Check sheet for the modelled part. Datum: model origin and axes. Units: mm. Face numbers are marked on the shaded views. Coordinates: 2 decimals unless noted, no trailing zeros. Loops run counter-clockwise (first coordinate to the right, second up) from the corner with the lowest first, then second, coordinate; pieces in that order, holes last. Notation, with made-up numbers: (47, 61.25) -> (102, 61.25) arc R15 ccw to (102, 79.25) -> close; hole circle Ø5 at (86, 3.5). An arc over 180 degrees is marked (long way). Use CSV: the item, a comma, the result in double quotes.
```python
from build123d import *
from OCP.BRepFilletAPI import BRepFilletAPI_MakeChamfer

# Parameters (mm, degrees)
BOSS_EXTRUDE1_DEPTH = 2.5
BOSS_EXTRUDE2_DEPTH = 5.5
CHAMFER2_SIZE       = 5.5
CHAMFER2_SIZE_2     = 0.192064232
CHAMFER3_SIZE       = 0.8
CHAMFER3_SIZE2      = 0.829452764


with BuildPart() as part:
    # Sketch1 → Boss-Extrude1 (new body)
    with BuildSketch(Plane(origin=(0, 0, 0), x_dir=(1, 0, 0), z_dir=(0, 1, 0))):
        with BuildLine():
            Line((-23, 17.5), (23, 17.5))
            ThreePointArc((23, 17.5), (28.656854249, 15.156854249), (31, 9.5))
            Line((31, 9.5), (31, -9.5))
            ThreePointArc((31, -9.5), (28.656854249, -15.156854249), (23, -17.5))
            Line((23, -17.5), (-23, -17.5))
            ThreePointArc((-23, -17.5), (-28.656854249, -15.156854249), (-31, -9.5))
            Line((-31, -9.5), (-31, 9.5))
            ThreePointArc((-31, 9.5), (-28.656854249, 15.156854249), (-23, 17.5))
        make_face()
    extrude(amount=BOSS_EXTRUDE1_DEPTH)

    # Sketch2 → Boss-Extrude2 (add)
    with BuildSketch(Plane(origin=(0, 2.5, 0), x_dir=(1, 0, 0), z_dir=(0, 1, 0))):
        with BuildLine():
            Line((-28.85, -7.8), (-28.85, 7.8))
            ThreePointArc((-28.85, 7.8), (-20.4, 16.25), (-11.95, 7.8))
            Line((-11.95, 7.8), (-11.95, -7.8))
            ThreePointArc((-11.95, -7.8), (-20.4, -16.25), (-28.85, -7.8))
        make_face()
        with BuildLine():
            Line((-8.45, -7.8), (-8.45, 7.8))
            ThreePointArc((-8.45, 7.8), (0, 16.25), (8.45, 7.8))
            Line((8.45, 7.8), (8.45, -7.8))
            ThreePointArc((8.45, -7.8), (0, -16.25), (-8.45, -7.8))
        make_face()
        with BuildLine():
            Line((11.95, -7.8), (11.95, 7.8))
            ThreePointArc((11.95, 7.8), (20.4, 16.25), (28.85, 7.8))
            Line((28.85, 7.8), (28.85, -7.8))
            ThreePointArc((28.85, -7.8), (20.4, -16.25), (11.95, -7.8))
        make_face()
    extrude(amount=BOSS_EXTRUDE2_DEPTH)

    # Chamfer2
    # the kernel refuses this chamfer: 5.5, 0.192064232 mm, written as the material it takes off along each edge
    with BuildSketch(Plane(origin=(-28.85, 8, 7.8), x_dir=(-0.0013423185755924486, -0.9999990990900149, 0), z_dir=(0, 0, -1))) as chamfer2_piece_1_section:
        Polygon((CHAMFER2_SIZE * 0.99999909909, -CHAMFER2_SIZE * 0.00134231857559), (-CHAMFER2_SIZE_2 * 0.00134231857702, -CHAMFER2_SIZE_2 * 0.999999100155), (0, 0), align=None)
    chamfer2_piece_1 = extrude(amount=15.6, mode=Mode.PRIVATE)
    chamfer2_piece_1 = split(chamfer2_piece_1, bisect_by=Plane(origin=(-28.848299171, 2.5, 0), z_dir=(0, 1, 0)), keep=Keep.TOP, mode=Mode.PRIVATE)
    add(chamfer2_piece_1, mode=Mode.SUBTRACT)
    with BuildSketch(Plane(origin=(-20.4, 8, -7.8), x_dir=(-1, 0, 0), z_dir=(0, 0, 1))) as chamfer2_piece_2_section:
        Polygon((8.45, CHAMFER2_SIZE), (8.45 - CHAMFER2_SIZE_2 * 1.00000000107, 0), (8.45, 0), align=None)
    chamfer2_piece_2 = revolve(axis=Axis((-20.4, 8, -7.8), (0, -1, 0)), revolution_arc=180, mode=Mode.PRIVATE)
    chamfer2_piece_2 = split(chamfer2_piece_2, bisect_by=Plane(origin=(-20.4, 2.5, -16.18152008), z_dir=(0, 1, 0)), keep=Keep.TOP, mode=Mode.PRIVATE)
    add(chamfer2_piece_2, mode=Mode.SUBTRACT)
    with BuildSketch(Plane(origin=(-11.95, 8, -7.8), x_dir=(0.0013423185755924486, -0.9999990990900149, 0), z_dir=(0, 0, 1))) as chamfer2_piece_3_section:
        Polygon((CHAMFER2_SIZE * 0.99999909909, -CHAMFER2_SIZE * 0.00134231857559), (-CHAMFER2_SIZE_2 * 0.00134231857702, -CHAMFER2_SIZE_2 * 0.999999100155), (0, 0), align=None)
    chamfer2_piece_3 = extrude(amount=15.6, mode=Mode.PRIVATE)
    chamfer2_piece_3 = split(chamfer2_piece_3, bisect_by=Plane(origin=(-11.951700829, 2.5, 0), z_dir=(0, 1, 0)), keep=Keep.TOP, mode=Mode.PRIVATE)
    add(chamfer2_piece_3, mode=Mode.SUBTRACT)
    with BuildSketch(Plane(origin=(-20.4, 8, 7.8), x_dir=(1, 0, 0), z_dir=(0, 0, -1))) as chamfer2_piece_4_section:
        Polygon((8.45, CHAMFER2_SIZE), (8.45 - CHAMFER2_SIZE_2 * 1.00000000107, 0), (8.45, 0), align=None)
    chamfer2_piece_4 = revolve(axis=Axis((-20.4, 8, 7.8), (0, -1, 0)), revolution_arc=180, mode=Mode.PRIVATE)
    chamfer2_piece_4 = split(chamfer2_piece_4, bisect_by=Plane(origin=(-20.4, 2.5, 16.18152008), z_dir=(0, 1, 0)), keep=Keep.TOP, mode=Mode.PRIVATE)
    add(chamfer2_piece_4, mode=Mode.SUBTRACT)
    with BuildSketch(Plane(origin=(-8.45, 8, 7.8), x_dir=(-0.0013423185755924486, -0.9999990990900149, 0), z_dir=(0, 0, -1))) as chamfer2_piece_5_section:
        Polygon((CHAMFER2_SIZE * 0.99999909909, -CHAMFER2_SIZE * 0.00134231857559), (-CHAMFER2_SIZE_2 * 0.00134231857702, -CHAMFER2_SIZE_2 * 0.999999100155), (0, 0), align=None)
    chamfer2_piece_5 = extrude(amount=15.6, mode=Mode.PRIVATE)
    chamfer2_piece_5 = split(chamfer2_piece_5, bisect_by=Plane(origin=(-8.448299171, 2.5, 0), z_dir=(0, 1, 0)), keep=Keep.TOP, mode=Mode.PRIVATE)
    add(chamfer2_piece_5, mode=Mode.SUBTRACT)
    with BuildSketch(Plane(origin=(0, 8, -7.8), x_dir=(-1, 0, 0), z_dir=(0, 0, 1))) as chamfer2_piece_6_section:
        Polygon((8.45, CHAMFER2_SIZE), (8.45 - CHAMFER2_SIZE_2 * 1.00000000107, 0), (8.45, 0), align=None)
    chamfer2_piece_6 = revolve(axis=Axis((0, 8, -7.8), (0, -1, 0)), revolution_arc=180, mode=Mode.PRIVATE)
    chamfer2_piece_6 = split(chamfer2_piece_6, bisect_by=Plane(origin=(0, 2.5, -16.18152008), z_dir=(0, 1, 0)), keep=Keep.TOP, mode=Mode.PRIVATE)
    add(chamfer2_piece_6, mode=Mode.SUBTRACT)
    with BuildSketch(Plane(origin=(8.45, 8, -7.8), x_dir=(0.0013423185755924486, -0.9999990990900149, 0), z_dir=(0, 0, 1))) as chamfer2_piece_7_section:
        Polygon((CHAMFER2_SIZE * 0.99999909909, -CHAMFER2_SIZE * 0.00134231857559), (-CHAMFER2_SIZE_2 * 0.00134231857702, -CHAMFER2_SIZE_2 * 0.999999100155), (0, 0), align=None)
    chamfer2_piece_7 = extrude(amount=15.6, mode=Mode.PRIVATE)
    chamfer2_piece_7 = split(chamfer2_piece_7, bisect_by=Plane(origin=(8.448299171, 2.5, 0), z_dir=(0, 1, 0)), keep=Keep.TOP, mode=Mode.PRIVATE)
    add(chamfer2_piece_7, mode=Mode.SUBTRACT)
    with BuildSketch(Plane(origin=(0, 8, 7.8), x_dir=(1, 0, 0), z_dir=(0, 0, -1))) as chamfer2_piece_8_section:
        Polygon((8.45, CHAMFER2_SIZE), (8.45 - CHAMFER2_SIZE_2 * 1.00000000107, 0), (8.45, 0), align=None)
    chamfer2_piece_8 = revolve(axis=Axis((0, 8, 7.8), (0, -1, 0)), revolution_arc=180, mode=Mode.PRIVATE)
    chamfer2_piece_8 = split(chamfer2_piece_8, bisect_by=Plane(origin=(0, 2.5, 16.18152008), z_dir=(0, 1, 0)), keep=Keep.TOP, mode=Mode.PRIVATE)
    add(chamfer2_piece_8, mode=Mode.SUBTRACT)
    with BuildSketch(Plane(origin=(11.95, 8, 7.8), x_dir=(-0.0013423185755924486, -0.9999990990900149, 0), z_dir=(0, 0, -1))) as chamfer2_piece_9_section:
        Polygon((CHAMFER2_SIZE * 0.99999909909, -CHAMFER2_SIZE * 0.00134231857559), (-CHAMFER2_SIZE_2 * 0.00134231857702, -CHAMFER2_SIZE_2 * 0.999999100155), (0, 0), align=None)
    chamfer2_piece_9 = extrude(amount=15.6, mode=Mode.PRIVATE)
    chamfer2_piece_9 = split(chamfer2_piece_9, bisect_by=Plane(origin=(11.951700829, 2.5, 0), z_dir=(0, 1, 0)), keep=Keep.TOP, mode=Mode.PRIVATE)
    add(chamfer2_piece_9, mode=Mode.SUBTRACT)
    with BuildSketch(Plane(origin=(20.4, 8, -7.8), x_dir=(-1, 0, 0), z_dir=(0, 0, 1))) as chamfer2_piece_10_section:
        Polygon((8.45, CHAMFER2_SIZE), (8.45 - CHAMFER2_SIZE_2 * 1.00000000107, 0), (8.45, 0), align=None)
    chamfer2_piece_10 = revolve(axis=Axis((20.4, 8, -7.8), (0, -1, 0)), revolution_arc=180, mode=Mode.PRIVATE)
    chamfer2_piece_10 = split(chamfer2_piece_10, bisect_by=Plane(origin=(20.4, 2.5, -16.18152008), z_dir=(0, 1, 0)), keep=Keep.TOP, mode=Mode.PRIVATE)
    add(chamfer2_piece_10, mode=Mode.SUBTRACT)
    with BuildSketch(Plane(origin=(28.85, 8, -7.8), x_dir=(0.0013423185755924486, -0.9999990990900149, 0), z_dir=(0, 0, 1))) as chamfer2_piece_11_section:
        Polygon((CHAMFER2_SIZE * 0.99999909909, -CHAMFER2_SIZE * 0.00134231857559), (-CHAMFER2_SIZE_2 * 0.00134231857702, -CHAMFER2_SIZE_2 * 0.999999100155), (0, 0), align=None)
    chamfer2_piece_11 = extrude(amount=15.6, mode=Mode.PRIVATE)
    chamfer2_piece_11 = split(chamfer2_piece_11, bisect_by=Plane(origin=(28.848299171, 2.5, 0), z_dir=(0, 1, 0)), keep=Keep.TOP, mode=Mode.PRIVATE)
    add(chamfer2_piece_11, mode=Mode.SUBTRACT)
    with BuildSketch(Plane(origin=(20.4, 8, 7.8), x_dir=(1, 0, 0), z_dir=(0, 0, -1))) as chamfer2_piece_12_section:
        Polygon((8.45, CHAMFER2_SIZE), (8.45 - CHAMFER2_SIZE_2 * 1.00000000107, 0), (8.45, 0), align=None)
    chamfer2_piece_12 = revolve(axis=Axis((20.4, 8, 7.8), (0, -1, 0)), revolution_arc=180, mode=Mode.PRIVATE)
    chamfer2_piece_12 = split(chamfer2_piece_12, bisect_by=Plane(origin=(20.4, 2.5, 16.18152008), z_dir=(0, 1, 0)), keep=Keep.TOP, mode=Mode.PRIVATE)
    add(chamfer2_piece_12, mode=Mode.SUBTRACT)

    # Chamfer3: one chamfer whose edges measure the first distance from different faces: ONE call of the kernel's chamfer builder (chamfer() names one face for all edges)
    chamfer3_edges_1 = [part.edges().sort_by_distance(p)[0] for p in [
        (-20.4, 8, 16.057935768),
    ]]
    chamfer3_side_1 = [part.faces().sort_by_distance(p)[0] for p in [
        (-20.4, 5.25, 16.153967884),
    ]]
    chamfer3_edges_2 = [part.edges().sort_by_distance(p)[0] for p in [
        (-12.142064232, 8, 0),
    ]]
    chamfer3_side_2 = [part.faces().sort_by_distance(p)[0] for p in [
        (-12.046032116, 5.25, 0),
    ]]
    chamfer3_edges_3 = [part.edges().sort_by_distance(p)[0] for p in [
        (-20.4, 8, -16.057935768),
    ]]
    chamfer3_side_3 = [part.faces().sort_by_distance(p)[0] for p in [
        (-20.4, 5.25, -16.153967884),
    ]]
    chamfer3_edges_4 = [part.edges().sort_by_distance(p)[0] for p in [
        (-28.657935768, 8, 0),
    ]]
    chamfer3_side_4 = [part.faces().sort_by_distance(p)[0] for p in [
        (-28.753967884, 5.25, 0),
    ]]
    chamfer3_edges_5 = [part.edges().sort_by_distance(p)[0] for p in [
        (0, 8, 16.057935768),
    ]]
    chamfer3_side_5 = [part.faces().sort_by_distance(p)[0] for p in [
        (0, 5.25, 16.153967884),
    ]]
    chamfer3_edges_6 = [part.edges().sort_by_distance(p)[0] for p in [
        (8.257935768, 8, 0),
    ]]
    chamfer3_side_6 = [part.faces().sort_by_distance(p)[0] for p in [
        (8.353967884, 5.25, 0),
    ]]
    chamfer3_edges_7 = [part.edges().sort_by_distance(p)[0] for p in [
        (0, 8, -16.057935768),
    ]]
    chamfer3_side_7 = [part.faces().sort_by_distance(p)[0] for p in [
        (0, 5.25, -16.153967884),
    ]]
    chamfer3_edges_8 = [part.edges().sort_by_distance(p)[0] for p in [
        (-8.257935768, 8, 0),
    ]]
    chamfer3_side_8 = [part.faces().sort_by_distance(p)[0] for p in [
        (-8.353967884, 5.25, 0),
    ]]
    chamfer3_edges_9 = [part.edges().sort_by_distance(p)[0] for p in [
        (20.4, 8, 16.057935768),
    ]]
    chamfer3_side_9 = [part.faces().sort_by_distance(p)[0] for p in [
        (20.4, 5.25, 16.153967884),
    ]]
    chamfer3_edges_10 = [part.edges().sort_by_distance(p)[0] for p in [
        (28.657935768, 8, 0),
    ]]
    chamfer3_side_10 = [part.faces().sort_by_distance(p)[0] for p in [
        (28.753967884, 5.25, 0),
    ]]
    chamfer3_edges_11 = [part.edges().sort_by_distance(p)[0] for p in [
        (20.4, 8, -16.057935768),
    ]]
    chamfer3_side_11 = [part.faces().sort_by_distance(p)[0] for p in [
        (20.4, 5.25, -16.153967884),
    ]]
    chamfer3_edges_12 = [part.edges().sort_by_distance(p)[0] for p in [
        (12.142064232, 8, 0),
    ]]
    chamfer3_side_12 = [part.faces().sort_by_distance(p)[0] for p in [
        (12.046032116, 5.25, 0),
    ]]
    chamfer3 = BRepFilletAPI_MakeChamfer(part.part.solid().wrapped)
    for e in chamfer3_edges_1:
        chamfer3.Add(CHAMFER3_SIZE, CHAMFER3_SIZE2, e.wrapped, chamfer3_side_1[0].wrapped)  # the first distance lies on this face
    for e in chamfer3_edges_2:
        chamfer3.Add(CHAMFER3_SIZE, CHAMFER3_SIZE2, e.wrapped, chamfer3_side_2[0].wrapped)  # the first distance lies on this face
    for e in chamfer3_edges_3:
        chamfer3.Add(CHAMFER3_SIZE, CHAMFER3_SIZE2, e.wrapped, chamfer3_side_3[0].wrapped)  # the first distance lies on this face
    for e in chamfer3_edges_4:
        chamfer3.Add(CHAMFER3_SIZE, CHAMFER3_SIZE2, e.wrapped, chamfer3_side_4[0].wrapped)  # the first distance lies on this face
    for e in chamfer3_edges_5:
        chamfer3.Add(CHAMFER3_SIZE, CHAMFER3_SIZE2, e.wrapped, chamfer3_side_5[0].wrapped)  # the first distance lies on this face
    for e in chamfer3_edges_6:
        chamfer3.Add(CHAMFER3_SIZE, CHAMFER3_SIZE2, e.wrapped, chamfer3_side_6[0].wrapped)  # the first distance lies on this face
    for e in chamfer3_edges_7:
        chamfer3.Add(CHAMFER3_SIZE, CHAMFER3_SIZE2, e.wrapped, chamfer3_side_7[0].wrapped)  # the first distance lies on this face
    for e in chamfer3_edges_8:
        chamfer3.Add(CHAMFER3_SIZE, CHAMFER3_SIZE2, e.wrapped, chamfer3_side_8[0].wrapped)  # the first distance lies on this face
    for e in chamfer3_edges_9:
        chamfer3.Add(CHAMFER3_SIZE, CHAMFER3_SIZE2, e.wrapped, chamfer3_side_9[0].wrapped)  # the first distance lies on this face
    for e in chamfer3_edges_10:
        chamfer3.Add(CHAMFER3_SIZE, CHAMFER3_SIZE2, e.wrapped, chamfer3_side_10[0].wrapped)  # the first distance lies on this face
    for e in chamfer3_edges_11:
        chamfer3.Add(CHAMFER3_SIZE, CHAMFER3_SIZE2, e.wrapped, chamfer3_side_11[0].wrapped)  # the first distance lies on this face
    for e in chamfer3_edges_12:
        chamfer3.Add(CHAMFER3_SIZE, CHAMFER3_SIZE2, e.wrapped, chamfer3_side_12[0].wrapped)  # the first distance lies on this face
    add(Compound.cast(chamfer3.Shape()), mode=Mode.REPLACE)


solid = part.part
```
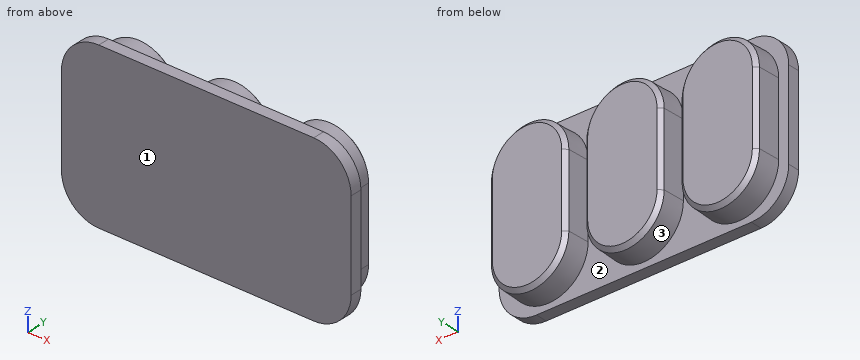
1) Cross-section at C-C on z = 5.5. Record the boundary of the cut face in (x, y), and give its area (3 significant figures).
Answer below:
outline,"(-31, 0) -> (31, 0) -> (31, 2.5) -> (28.85, 2.5) -> (28.69, 7.2) -> (27.83, 8) -> (12.97, 8) -> (12.11, 7.2) -> (11.95, 2.5) -> (8.45, 2.5) -> (8.29, 7.2) -> (7.43, 8) -> (-7.43, 8) -> (-8.29, 7.2) -> (-8.45, 2.5) -> (-11.95, 2.5) -> (-12.11, 7.2) -> (-12.97, 8) -> (-27.83, 8) -> (-28.69, 7.2) -> (-28.85, 2.5) -> (-31, 2.5) -> close"
area,"429 mm²"
2) Draft check along X on the marked faces 1, 2 and 3. Enter one of: released by +X, released by -X, zero draft, split by the parting line, or undercut.
Answer below:
face 1,"zero draft"
face 2,"undercut"
face 3,"undercut"
3) Cross-section at D-D on x = 0. Record the boundary of the cut face in (y, z), and give its area (3 significant figures).
Answer below:
outline,"(0, -17.5) -> (2.5, -17.5) -> (2.5, -16.25) -> (7.2, -16.09) -> (8, -15.23) -> (8, 15.23) -> (7.2, 16.09) -> (2.5, 16.25) -> (2.5, 17.5) -> (0, 17.5) -> close"
area,"265 mm²"
4) Go/stop test with flat-tipped pins: pin 1 Ø1.5 at (x, y) = (15, 7) entering from -Z; pin 2 Ø4 at (x, y) = (-11, 6.5) entering from +Z; pin 3 Ø4 at (x, y) = (22, 6.5) entering from +Z. Record where each tip stops, or that it passes through.
Answer below:
pin 1,"stops at z = -14.67"
pin 2,"stops at z = 11.58"
pin 3,"stops at z = 16.16"
5) Cross-section at B-B on y = 5.75. Record the boundary of the cut face in (x, z), and give its area (3 significant figures).
Answer below:
outline,"(-28.74, -7.8) arc R8.34 ccw to (-12.06, -7.8) -> (-12.06, 7.8) arc R8.34 ccw to (-28.74, 7.8) -> close; (-8.34, -7.8) arc R8.34 ccw to (8.34, -7.8) -> (8.34, 7.8) arc R8.34 ccw to (-8.34, 7.8) -> close; (12.06, -7.8) arc R8.34 ccw to (28.74, -7.8) -> (28.74, 7.8) arc R8.34 ccw to (12.06, 7.8) -> close"
area,"1,440 mm²"
6) Cross-section at A-A on y = 1.75. Record the boundary of the cut face in (x, z), and give its area (3 significant figures).
Answer below:
outline,"(-31, -9.5) arc R8 ccw to (-23, -17.5) -> (23, -17.5) arc R8 ccw to (31, -9.5) -> (31, 9.5) arc R8 ccw to (23, 17.5) -> (-23, 17.5) arc R8 ccw to (-31, 9.5) -> close"
area,"2,120 mm²"
7) Thickness scan on line 1 along X through (y, z) = (5.25, 9); line 2 along X through (y, z) = (4.5, 13.5); line 3 along Y through (x, z) = (-7, 13). Record the ranges inside material, lowest first. Write a range as from..to.
Answer below:
line 1,"x = -28.67..-12.13, -8.27..8.27, 12.13..28.67"
line 2,"x = -26.54..-14.26, -6.14..6.14, 14.26..26.54"
line 3,"y = 0..2.5"
